Verification items for the finished model (mm, model axes). Face numbers are marked on the shaded views. A direction names the side the tool comes from. Give positions to 0.01 mm unless a question says otherwise; leave off trailing zeros. Write each loop counter-clockwise with the first axis right and the second up, starting at its lowest first coordinate (ties: lowest second). Pieces come first, ordered by that corner, then holes. Notation, with made-up numbers: (35.25, -40) -> (42.25, -40) arc R21 ccw to (42.25, -3) -> close; hole circle Ø7 at (45, 56.25). An arc over 180 degrees is marked (long way). Answer as CSV lines item,"result". Start each with the question number.
1) Sectioned sample at D-D on y = -9. Record the cut outline in (x, z).
2) Tool access check on the marked faces 5, 6, 7, 8 and 9. Record the directions out of +Z, -Z, +X, -X, +Y, -Y that give a thin tool (end or side, any length) a straight path to the whole face; none if there is none.
3) Material ranges on L1, parallel to Z at x = 5.25, y = -5; L2, parallel to Y at x = 9.15, z = -6; L3, parallel to X at y = -7, z = 1.25, recorded low to high.
4) Mould release check, pull along Y, two halves, no side actions. Record for the marked faces 1, 2, 3 and 4: released by +Y, released by -Y, zero draft, split by the parting line, or undercut.
5) Sectioned sample at A-A on x = 5. Record the cut outline in (y, z).
6) Sectioned sample at B-B on z = -6. Record the cut outline in (x, y).
7) Sectioned sample at C-C on z = 1.75. Record the cut outline in (x, y), and give its area (3 significant figures).
8) Gauge pin test, flat ends, axial feed: pin 1 Ø2 at (x, z) = (4, 8) entering from -Y; pin 2 Ø1.5 at (x, z) = (5.5, -3) entering from +Y; pin 3 Ø5 at (x, y) = (6.5, -7) entering from -Z. Record the tip position at first contact, or that the pin passes through.
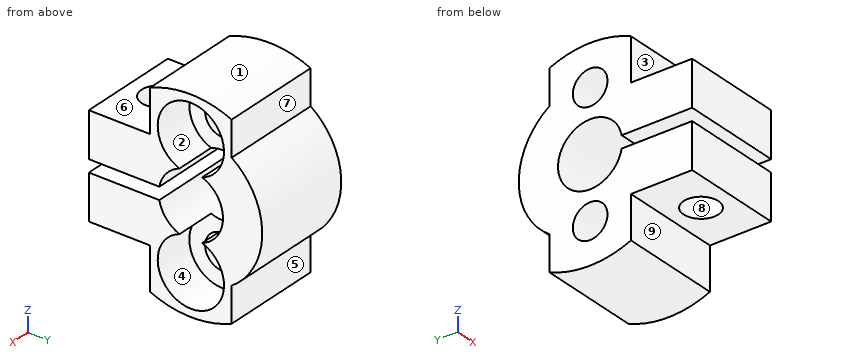
Autodesk Inventor part; units mm, degrees
ref_plane "YZ Plane" through (0, 0, 0) normal (1, 0, 0) x (0, 1, 0)
ref_plane "XZ Plane" through (0, 0, 0) normal (0, 1, 0) x (-1, 0, 0)
ref_plane "XY Plane" through (0, 0, 0) normal (0, 0, 1) x (1, 0, 0)
sketch "スケッチ1" plane through (0, 0, 0) normal (1, 0, 0) x (0, 1, 0)
  circle A0 centre (0, 0) radius 3.15
  circle A1 centre (0, 0) radius 7
  line L0 (0, 5) -> (-10, 5)
  line L1 (-10, 5) -> (-10, -5)
  line L2 (-10, -5) -> (0, -5)
  line L3 (0, -5) -> (0, 5) construction
  line L4 (-10, 0.6) -> (0, 0.6)
  line L5 (0, 0.6) -> (0, -0.6)
  line L6 (0, -0.6) -> (-10, -0.6)
  line L7 (-10, -0.6) -> (-10, 0.6)
  line L8 (4, 10) -> (-4, 10) construction
  line L9 (-4, 10) -> (-4, -10)
  line L10 (-4, -10) -> (4, -10) construction
  line L11 (4, -10) -> (4, 10)
  line L12 (4, 10) -> (-4, -10) construction
  line L13 (-4, 10) -> (4, -10) construction
  arc A2 (4, 9.1652) -> (-4, 9.1652) centre (0, 0) ccw
  arc A3 (-4, -9.1652) -> (4, -9.1652) centre (0, 0) ccw
  point P0 (-11, 3.3541)
  point P1 (-11, -3.3541)
  point P2 (-4.899, 5)
  point P3 (-4.899, -5)
  point P4 (-3.0923, 0.6)
  point P5 (-3.0923, -0.6)
  point P6 (-6.9742, -0.6)
  point P7 (-6.9742, 0.6)
  point P8 (0, -3.15)
  point P9 (0, 3.15)
  point P10 (0, 0.6)
  point P11 (-4, -5)
  point P12 (4, -5.7446)
  point P13 (4, 5.7446)
  point P14 (-4, 5)
  dimension "d0" = 6.3
  dimension "d1" = 14
  dimension "d2" = 5
  dimension "d3" = 5
  dimension "d4" = 10
  dimension "d18" = 1.2
  dimension "d19" = 0.6
  dimension "d45" = 8
  dimension "d46" = 20
extrude "押し出し1" add sketch "スケッチ1" along normal blind 10 contours A0 L4 L9 A1 L11 L6 | L4 A1 L0 L9 | L9 L2 A1 L6 | L4 L1 L0 A1 | A1 L2 L1 L6 | L9 A2 L11 A1 | A1 L11 A3 L9 | A1 L11
sketch "スケッチ2" plane through (10, 0, 0) normal (1, 0, 0) x (0, 0, -1)
  line L0 (14, 0) -> (-14, 0)
  point P0 (0, 0)
  point P1 (-6, 0)
  point P2 (6, 0)
  dimension "d7" = 6
  dimension "d8" = 6
hole "穴1" at (10, 0, 6) at (10, 0, -6) direction (-1, 0, 0) diameter 3.4 end through all counterbore diameter 6.5 counterbore depth 4
sketch "スケッチ3" plane through (0, -4.899, 5) normal (0, 0, 1) x (1, 0, 0)
  line L0 (0, -5.101) -> (10, -5.101)
  point P0 (5, -2.101)
  point P1 (5, -5.101)
  dimension "d44" = 3
hole "穴2" at (5, -7, 5) direction (0, 0, -1) diameter 3.4 end through all
properties part number "セットカラ―" material "ABS プラスチック"
Ans:
1,outline,"(0, -5) -> (10, -5) -> (10, -0.6) -> (0, -0.6) -> close; (0, 0.6) -> (10, 0.6) -> (10, 5) -> (0, 5) -> close"
2,face 5,"-Z, +X, -X, +Y"
2,face 6,"+Z, +X, -X, -Y"
2,face 7,"+Z, +X, -X, +Y"
2,face 8,"+Z, -Z"
2,face 9,"-Z, +X, -X, -Y"
3,L1,"z = -5 to -0.6, 0.6 to 5"
3,L2,"y = -4 to -3.25, 3.25 to 4"
3,L3,"x = 0 to 3.3, 6.7 to 10"
4,face 1,"split by the parting line"
4,face 2,"undercut"
4,face 3,"released by -Y"
4,face 4,"undercut"
5,outline,"(-10, -5) -> (-8.7, -5) -> (-8.7, -0.6) -> (-10, -0.6) -> close; (-10, 0.6) -> (-8.7, 0.6) -> (-8.7, 5) -> (-10, 5) -> close; (-5.3, -5) -> (-4, -5) -> (-4, -9.17) arc R10 ccw to (4, -9.17) -> (4, -5.74) arc R7 ccw to (4, 5.74) -> (4, 9.17) arc R10 ccw to (-4, 9.17) -> (-4, 5) -> (-5.3, 5) -> (-5.3, 0.6) -> (-3.09, 0.6) arc R3.15 cw (long way) to (-3.09, -0.6) -> (-5.3, -0.6) -> close; hole circle Ø3.4 at (0, -6); hole circle Ø3.4 at (0, 6)"
6,outline,"(0, -4) -> (10, -4) -> (10, -3.25) -> (6, -3.25) -> (6, -1.7) -> (0, -1.7) -> close; (0, 1.7) -> (6, 1.7) -> (6, 3.25) -> (10, 3.25) -> (10, 4) -> (0, 4) -> close"
7,outline,"(0, -10) -> (10, -10) -> (10, -2.62) -> (0, -2.62) -> close; (0, 2.62) -> (10, 2.62) -> (10, 6.78) -> (0, 6.78) -> close; hole circle Ø3.4 at (5, -7)"
7,area,"106 mm²"
8,pin 1,"stops at y = -4"
8,pin 2,"stops at y = 6.63"
8,pin 3,"stops at z = -5"
